Check sheet for the modelled part. Datum: model origin and axes. Units: mm. A direction names the side the tool comes from. Give positions to 0.01 mm unless a question says otherwise; leave off trailing zeros. Loops run counter-clockwise (first coordinate to the right, second up) from the corner with the lowest first, then second, coordinate; pieces in that order, holes last. Notation, with made-up numbers: (81.25, 0) -> (88.25, 0) arc R7 ccw to (88.25, 7) -> close; hole circle Ø1 at (28, 62.5). An arc over 180 degrees is marked (long way). Write each question's results on one line, items separated by ' | '. Start each with the question number.
Item 1: Scan lines: line 1 along Y through (x, z) = (-3.5, 0) (1 decimal); line 2 along Z through (x, y) = (-3.5, 2.54) (1 decimal); line 3 along X through (y, z) = (5.5, 1). Record each from-to range of solid material in increasing order.
Item 2: Cross-section at C-C on z = 7.5. Enter the section's corners in (x, y) (3 decimals).
Item 3: Gauge pin test, flat ends, axial feed: pin 1 Ø5 at (x, y) = (3.5, 6) entering from -Z; pin 2 Ø4 at (x, z) = (6, 4) entering from +Y; pin 3 Ø1.5 at (y, z) = (11, -3) entering from +X. Record the tip position at first contact, or that the pin passes through.
Item 4: Cross-section at D-D on y = -2. Enter the section's corners in (x, z) (1 decimal).
Item 5: Mould release check, pull along X, two halves, no side actions. Record for faces 1 (the face through (0, 0, 0)), 2 (the face through (6.957, -1.61, 7.059)), 3 (the face through (-2.704, 0.254, 4.712)), 4 (the face through (-9.208, 5, 0)): pulls with the +X half, pulls with the -X half, needs draft (parallel to the pull), parting line crosses it, or undercut.
Item 6: Cross-section at B-B on x = -8. Enter the section's corners in (y, z) (1 decimal), then the cut area to 3 significant figures.
Item 7: Access from +Z, -Z, +X, -X, +Y, -Y to the whole of each face (thin tool, end or side, straight path). Record for faces 5 (the face through (0, -2, 11.049)), 6 (the face through (2.08, 6.01, -0.27)), 7 (the face through (-4.445, -2, 8)).
from build123d import *

# Parameters (mm, degrees)
SKETCH1_R           = 4.445
SKETCH1_R_2         = 2.0955
BOSS_EXTRUDE1_DEPTH = 12.7
BOSS_EXTRUDE2_START = 3.175
SKETCH2_R           = 1.6256
BOSS_EXTRUDE2_DEPTH = 3.175
FILLET5_R           = 1.27
BOSS_EXTRUDE3_REACH = 24.275
CHAMFER1_SIZE       = 0.508
SKETCH3_R           = 2.2225
CUT_EXTRUDE1_DEPTH  = 8.255
FILLET6_R           = 0.889


with BuildPart() as part:
    # Sketch1 → Boss-Extrude1 (new body)
    with BuildSketch(Plane(origin=(0, 0, 0), x_dir=(1, 0, 0), z_dir=(0, 1, 0))):
        with Locations(Location((0, 0, 0), (0, 0, 270))):
            Circle(SKETCH1_R)
        with Locations(Location((0, 0, 0), (0, 0, 270))):
            Circle(SKETCH1_R_2, mode=Mode.SUBTRACT)
    extrude(amount=BOSS_EXTRUDE1_DEPTH)

    # Sketch2 → Boss-Extrude2 (add)
    with BuildSketch(Plane.XZ.offset(BOSS_EXTRUDE2_START)):
        with BuildLine():
            Line((-4.445, 0), (-4.445, 11.049))
            Line((-4.445, 11.049), (2.966769491, 11.049))
            Line((2.966769491, 11.049), (11.049, 2.966769491))
            Line((11.049, 2.966769491), (11.049, -4.445))
            Line((11.049, -4.445), (0, -4.445))
            ThreePointArc((0, -4.445), (-3.143089642, -3.143089642), (-4.445, 0))
        make_face()
        with Locations(Location((0, 7.62, 0), (0, 0, 270))):
            Circle(SKETCH2_R, mode=Mode.SUBTRACT)
        with Locations(Location((7.62, 0, 0), (0, 0, 270))):
            Circle(SKETCH2_R, mode=Mode.SUBTRACT)
    extrude(amount=-BOSS_EXTRUDE2_DEPTH)

    # Fillet5
    fillet5_edges = [part.edges().sort_by_distance(p)[0] for p in [
        (11.049, -1.5875, -4.445),
        (11.049, -1.5875, 2.966769491),
        (2.966769491, -1.5875, 11.049),
        (-4.445, -1.5875, 11.049),
    ]]
    fillet(fillet5_edges, radius=FILLET5_R)

    # Boss-Extrude3: up to this face of the body (flat: up to its plane)
    boss_extrude3_end = Plane(part.part.faces().sort_by_distance((2.521124126, -3.175, 2.521124126))[0])
    # Sketch4 → Boss-Extrude3 (add, up to the picked face)
    with BuildSketch(Plane(origin=(0, 12.7, 0), x_dir=(1, 0, 0), z_dir=(0, 1, 0)), mode=Mode.PRIVATE) as boss_extrude3_sk1:
        with BuildLine():
            Line((0, 4.445), (-9.2075, 4.445))
            Line((-9.2075, 4.445), (-9.2075, -4.445))
            Line((-9.2075, -4.445), (0, -4.445))
            ThreePointArc((0, -4.445), (-4.445, 0), (0, 4.445))
        make_face()
    boss_extrude3_tool1 = split(extrude(boss_extrude3_sk1.sketch, amount=-BOSS_EXTRUDE3_REACH, mode=Mode.PRIVATE), bisect_by=boss_extrude3_end, keep=Keep.BOTH, mode=Mode.PRIVATE)
    add(boss_extrude3_tool1.solids().sort_by(Axis((-6.263205, 12.7, 0), (0, -1, 0)))[0])

    # Chamfer1
    chamfer1_edges = [part.edges().sort_by_distance(p)[0] for p in [
        (0, 12.7, -2.0955),
    ]]
    chamfer(chamfer1_edges, length=CHAMFER1_SIZE)

    # Sketch3 → Cut-Extrude1 (cut)
    with BuildSketch(Plane(origin=(-9.2075, 0, 0), x_dir=(0, 0, -1), z_dir=(1, 0, 0))):
        with Locations(Location((0, 8.89, 0), (0, 0, 212.878349564))):
            Circle(SKETCH3_R)
        with Locations(Location((0, 2.54, 0), (0, 0, 212.878349564))):
            Circle(SKETCH3_R)
    extrude(amount=CUT_EXTRUDE1_DEPTH, mode=Mode.SUBTRACT)

    # Fillet6
    # the kernel refuses this fillet: 0.889 mm, written as the material it adds along each edge
    with BuildSketch(Plane(origin=(-4.445, 0, 4.445), x_dir=(-1, 0, 0), z_dir=(0, -1, 0))) as fillet6_piece_1:
        with BuildLine():
            CenterArc((FILLET6_R, -FILLET6_R), FILLET6_R, 90, 90)
            Line((0, -FILLET6_R), (0, 0))
            Line((0, 0), (FILLET6_R, 0))
        make_face()
    extrude(amount=3.175)
    with BuildSketch(Plane(origin=(0, 0, 0), x_dir=(0, 0, 1), z_dir=(-1, 0, 0))) as fillet6_piece_2_section:
        with BuildLine():
            CenterArc((4.445 + FILLET6_R, FILLET6_R), FILLET6_R, 180, 90)
            Line((4.445 + FILLET6_R, 0), (4.445, 0))
            Line((4.445, 0), (4.445, FILLET6_R))
        make_face()
    fillet6_piece_2 = revolve(axis=Axis((0, 0, 0), (0, 1, 0)), revolution_arc=228.779733666, mode=Mode.PRIVATE)
    fillet6_piece_2 = split(fillet6_piece_2, bisect_by=Plane(origin=(0, 0, -4.445), z_dir=(0, 0, 1)), keep=Keep.TOP, mode=Mode.PRIVATE)
    add(fillet6_piece_2)
    with BuildSketch(Plane(origin=(-4.445, 0, 4.445), x_dir=(0, 1, 0), z_dir=(1, 0, 0))) as fillet6_piece_3:
        with BuildLine():
            CenterArc((FILLET6_R, FILLET6_R), FILLET6_R, 180, 90)
            Line((0, FILLET6_R), (0, 0))
            Line((0, 0), (FILLET6_R, 0))
        make_face()
    extrude(amount=4.445)
    with BuildSketch(Plane(origin=(-6.6675, 0, 4.445), x_dir=(0, 1, 0), z_dir=(1, 0, 0))) as fillet6_piece_4a_section:
        with BuildLine():
            CenterArc((FILLET6_R, FILLET6_R), FILLET6_R, 180, 90)
            Line((0, FILLET6_R), (0, 0))
            Line((0, 0), (FILLET6_R, 0))
        make_face()
    fillet6_piece_4a = extrude(amount=6.6675, mode=Mode.PRIVATE)
    fillet6_piece_4a = split(fillet6_piece_4a, bisect_by=Plane(origin=(-4.445, 0, 4.445), z_dir=(-1, 0, 0)), keep=Keep.TOP, mode=Mode.PRIVATE)
    with BuildSketch(Plane(origin=(-4.445, 2.2225, 4.445), x_dir=(-1, 0, 0), z_dir=(0, -1, 0))) as fillet6_piece_4b_section:
        with BuildLine():
            CenterArc((FILLET6_R, -FILLET6_R), FILLET6_R, 90, 90)
            Line((0, -FILLET6_R), (0, 0))
            Line((0, 0), (FILLET6_R, 0))
        make_face()
    fillet6_piece_4b = extrude(amount=5.3975, mode=Mode.PRIVATE)
    fillet6_piece_4b = split(fillet6_piece_4b, bisect_by=Plane(origin=(-4.445, 0, 4.445), z_dir=(0, 1, 0)), keep=Keep.TOP, mode=Mode.PRIVATE)
    fillet6_piece_4 = fillet6_piece_4a & fillet6_piece_4b
    add(fillet6_piece_4)


solid = part.part
Answer sheet:
1) line 1: y = -3.2 to 0.3, 4.8 to 6.7, 11.1 to 12.7 | line 2: z = -4.4 to -2.2, 2.2 to 4.4 | line 3: x = -9.21 to -1.84, 1.84 to 4.33
2) outline: (-4.445, -3.175) -> (-1.621, -3.175) -> (-1.621, 0) -> (-4.445, 0) -> close; (1.621, -3.175) -> (6.516, -3.175) -> (6.516, 0) -> (1.621, 0) -> close
3) pin 1: stops at z = -4.33 | pin 2: stops at y = 0.01 | pin 3: stops at x = 3.83
4) outline: (-9.2, -4.4) -> (9.8, -4.4) arc R1.3 ccw to (11, -3.2) -> (11, 2.4) arc R1.3 ccw to (10.7, 3.3) -> (3.3, 10.7) arc R1.3 ccw to (2.4, 11) -> (-3.2, 11) arc R1.3 ccw to (-4.4, 9.8) -> (-4.4, 5.3) arc R0.9 cw to (-5.3, 4.4) -> (-9.2, 4.4) -> close; hole circle Ø3.3 at (0, 7.6); hole circle Ø3.3 at (7.6, 0)
5) face 1: undercut | face 2: pulls with the +X half | face 3: needs draft | face 4: pulls with the -X half
6) outline: (-3.2, -4.4) -> (12.7, -4.4) -> (12.7, 4.4) -> (-3.2, 4.4) -> close; hole circle Ø4.4 at (2.5, 0); hole circle Ø4.4 at (8.9, 0) | area: 110 mm²
7) face 5: +Z, +X, -X, +Y, -Y | face 6: +Y | face 7: +Z, -X, +Y, -Y
